from build123d import *

# Parameters (mm, degrees)
BOSS_EXTRUDE1_DEPTH      = 130
FILLET1_R                = 20
BOSS_EXTRUDE2_DEPTH      = 90
BOSS_EXTRUDE2_DEPTH_BACK = 200
SKETCH2_R                = 10
FILLET2_R                = 10


with BuildPart() as part:
    # Sketch1 → Boss-Extrude1 (new body)
    with BuildSketch(Plane(origin=(0, 0, 0), x_dir=(0, 0, -1), z_dir=(1, 0, 0))):
        with BuildLine():
            Line((-58.27789047, 15.260561771), (-90.331379838, 15.260561771))
            Line((-90.331379838, 15.260561771), (-90.331379838, -15.260561771))
            Line((-90.331379838, -15.260561771), (-58.27789047, -15.260561771))
            ThreePointArc((-58.27789047, -15.260561771), (60.242819184, 0), (-58.27789047, 15.260561771))
        make_face()
        with BuildLine():
            ThreePointArc((-9.539392014, -3), (10, 0), (-9.539392014, 3))
            ThreePointArc((-9.539392014, 3), (-10, 0), (-9.539392014, -3))
        make_face(mode=Mode.SUBTRACT)
    extrude(amount=BOSS_EXTRUDE1_DEPTH)

    # Fillet1
    fillet1_edges = [part.edges().sort_by_distance(p)[0] for p in [
        (65, -15.260561771, 58.27789047),
        (65, 15.260561771, 58.27789047),
    ]]
    fillet(fillet1_edges, radius=FILLET1_R)

    # Sketch2 → Boss-Extrude2 (add, two sides: drawn at the far end of the back side and taken through both)
    with BuildSketch(Plane.ZY.offset(-BOSS_EXTRUDE2_DEPTH_BACK)):
        Circle(SKETCH2_R)
    extrude(amount=BOSS_EXTRUDE2_DEPTH + BOSS_EXTRUDE2_DEPTH_BACK)

    # Fillet2
    fillet2_edges = [part.edges().sort_by_distance(p)[0] for p in [
        (130, 0, -10),
        (0, 0, -10),
    ]]
    fillet(fillet2_edges, radius=FILLET2_R)


solid = part.part
Work out the finished part from the listing and answer in its coordinate system (mm). A direction names the side the tool comes from. Give positions to 0.01 mm unless a question says otherwise; leave off trailing zeros. Loops run counter-clockwise (first coordinate to the right, second up) from the corner with the lowest first, then second, coordinate; pieces in that order, holes last. Notation, with made-up numbers: (74.5, 76) -> (104.5, 76) arc R27 ccw to (104.5, 96) -> close; hole circle Ø7 at (-32, 80). An arc over 180 degrees is marked (long way). Use a Markdown table: item, result. Add a question column.
1) Each of these flat-tipped pins is pushed along its axis until it touches: P1, Ø5, axis at y = 39, z = -36, coming from the -X side; P2, Ø5, axis at x = 15.5, y = -38.5, coming from the +Z side; P3, Ø1.5, axis at x = -9, y = 3.5, coming from the +Z side; P4, Ø3, axis at x = -2.5, z = 60, coming from the -Y side. Where does it stop, or does it pass through?
2) The part is cut by section C-C, the plane z = 26. Determine the outline of the cut face in (x, y).
3) Consider line 1 along Z through (x, y) = (34.5, -1); line 2 along X through (y, z) = (43, 32); line 3 along Y through (x, z) = (65.5, -19). Determine where each line is inside the solid, lowest interval first.
4) The part is cut by section A-A, the plane x = 31.5. Determine the outline of the cut face in (y, z), plus the area to 3 significant figures.
5) The part is cut by section B-B, the plane y = 49. Determine the outline of the cut face in (x, z), plus the area to 3 significant figures.
6) Which of the six approach directions +Z, -Z, +X, -X, +Y, -Y give full straight-line access (tool end or side, diameter ignored) to faces 1 (the cylindrical face through (-49.44, -9.76, -2.17)), 2 (the cylindrical face through (170.42, -9.76, -2.17)), 3 (the flat face through (64, 15.261, 81)), 4 (the flat face through (64, -15.261, 81))?
Reported:
| question | item | result |
|---|---|---|
| 1 | P1 | stops at x = 0 |
| 1 | P2 | stops at z = 48.3 |
| 1 | P3 | stops at z = 9.68 |
| 1 | P4 | passes through |
| 2 | outline | (0, -54.34) -> (130, -54.34) -> (130, 54.34) -> (0, 54.34) -> close |
| 3 | line 1 | z = -60.23 to 90.33 |
| 3 | line 2 | x = 0 to 130 |
| 3 | line 3 | y = -57.17 to 57.17 |
| 4 | outline | (-26.47, 54.11) arc R60.24 ccw (long way) to (26.47, 54.11) arc R20 cw to (15.26, 72.08) -> (15.26, 90.33) -> (-15.26, 90.33) -> (-15.26, 72.08) arc R20 cw to start |
| 4 | area | 12,400 mm^2 |
| 5 | outline | (0, -35.05) -> (130, -35.05) -> (130, 35.05) -> (0, 35.05) -> close |
| 5 | area | 9,110 mm^2 |
| 6 | face 1 | -X |
| 6 | face 2 | +X |
| 6 | face 3 | +Z, +X, -X, +Y |
| 6 | face 4 | +Z, +X, -X, -Y |
